```python
from build123d import *

# Parameters (mm, degrees)
SKETCH_1_R          = 1.35
EXTRUDE_1_DEPTH     = 40
EXTRUDE_2_DEPTH     = 10
SKETCH_3_W          = 36
SKETCH_3_H          = 37.441664415
SKETCH_3_R          = 11
EXTRUDE_3_DEPTH     = 5
SKETCH_4_R          = 1.8
CUT_EXTRUDE_1_DEPTH = 18
SKETCH_5_R          = 1.35
CUT_EXTRUDE_2_DEPTH = 18
CUT_EXTRUDE_START   = -5
SKETCH_6_R          = 11
CUT_EXTRUDE_3_DEPTH = 5
SKETCH_7_W          = 36
SKETCH_7_H          = 37.441664415
CUT_EXTRUDE_4_DEPTH = 5
CUT_EXTRUDE_START_2 = -12
SKETCH_8_R          = 1.35
CUT_EXTRUDE_5_DEPTH = 12
SKETCH_10_R         = 1.34
SKETCH_10_R_2       = 1.35
CUT_EXTRUDE_6_DEPTH = 8


with BuildPart() as part:
    # 草图1 → 凸台-拉伸1 (new body)
    with BuildSketch(Plane.XY):
        with BuildLine():
            Line((-10, -4), (10, -4))
            ThreePointArc((10, -4), (13.795550466, -1.262456597), (12.395858862, 3.203101671))
            Line((12.395858862, 3.203101671), (6.347732719, 7.726984491))
            Line((6.347732719, 7.726984491), (0, 7.726984491))
            Line((0, 7.726984491), (-6.347732719, 7.726984491))
            Line((-6.347732719, 7.726984491), (-12.395858862, 3.203101671))
            ThreePointArc((-12.395858862, 3.203101671), (-13.795550466, -1.262456597), (-10, -4))
        make_face()
        with Locations((10, 0)):
            Circle(SKETCH_1_R, mode=Mode.SUBTRACT)
        with Locations((-10, 0)):
            Circle(SKETCH_1_R, mode=Mode.SUBTRACT)
    extrude(amount=EXTRUDE_1_DEPTH)

    # 草图2 → 凸台-拉伸2 (add)
    with BuildSketch(Plane.XZ.offset(4)):
        Polygon((-10, 37.441664415), (-18, 37.441664415), (-18, 0), (0, 0), (10, 0), (18, 0), (18, 37.441664415), align=None)
    extrude(amount=-EXTRUDE_2_DEPTH)

    # 草图3 → 凸台-拉伸3 (add)
    with BuildSketch(Plane.XZ.offset(4)):
        with Locations((0, 18.720832208)):
            Rectangle(SKETCH_3_W, SKETCH_3_H)
        with Locations(Location((0, 16, 0), (0, 0, 270))):
            Circle(SKETCH_3_R, mode=Mode.SUBTRACT)
    extrude(amount=EXTRUDE_3_DEPTH)

    # 草图4 → 切除-拉伸1 (cut)
    with BuildSketch(Plane.XZ.offset(4)):
        with Locations(Location((0, 16, 0), (0, 0, 270))):
            Circle(SKETCH_4_R)
    extrude(amount=-CUT_EXTRUDE_1_DEPTH, mode=Mode.SUBTRACT)

    # 草图5 → 切除-拉伸2 (cut)
    with BuildSketch(Plane.XZ.offset(9)):
        with Locations(Location((-15, 16, 0), (0, 0, 270))):
            Circle(SKETCH_5_R)
        with Locations(Location((15, 16, 0), (0, 0, 270))):
            Circle(SKETCH_5_R)
    extrude(amount=-CUT_EXTRUDE_2_DEPTH, mode=Mode.SUBTRACT)

    # 草图6 → 切除-拉伸3 (cut)
    with BuildSketch(Plane.XZ.offset(4).offset(CUT_EXTRUDE_START)):
        with Locations(Location((0, 16, 0), (0, 0, 270))):
            Circle(SKETCH_6_R)
    extrude(amount=CUT_EXTRUDE_3_DEPTH, mode=Mode.SUBTRACT)

    # 草图7 → 切除-拉伸4 (cut)
    with BuildSketch(Plane.XZ.offset(9)):
        with Locations((0, 18.720832208)):
            Rectangle(SKETCH_7_W, SKETCH_7_H)
    extrude(amount=-CUT_EXTRUDE_4_DEPTH, mode=Mode.SUBTRACT)

    # 草图8 → 切除-拉伸5 (cut)
    with BuildSketch(Plane.XY.offset(37.441664415).offset(CUT_EXTRUDE_START_2)):
        with Locations((10, 0)):
            Circle(SKETCH_8_R)
        with Locations((-10, 0)):
            Circle(SKETCH_8_R)
    extrude(amount=CUT_EXTRUDE_5_DEPTH, mode=Mode.SUBTRACT)

    # 草图10 → 切除-拉伸6 (cut)
    with BuildSketch(Plane(origin=(0, 0, 0), x_dir=(-1, 0, 0), z_dir=(0, 0, -1))):
        with Locations((10, 0)):
            Circle(SKETCH_10_R)
        with Locations(Location((-10, 0, 0), (0, 0, 180))):
            Circle(SKETCH_10_R_2)
    extrude(amount=-CUT_EXTRUDE_6_DEPTH, mode=Mode.SUBTRACT)


solid = part.part
```
Here's how the part is built. I have some questions about the finished solid (model axes, mm). A direction names the side the tool comes from. Give positions to 0.01 mm unless a question says otherwise; leave off trailing zeros. Order: outer loops, then holes, each group sorted by start corner. A loop starts at its lowest first (then second) coordinate and runs counter-clockwise, first axis right, second up. Notation, with made-up numbers: (19, 50) -> (28, 50) arc R21 cw to (28, 79) -> close; hole circle Ø7 at (75.5, 72.5). An arc over 180 degrees is marked (long way). Use CSV: the item, a comma, the result in double quotes. Start each with the question number.
Item 1: Suppose I cut it at C-C (z = 30.5). List the corners of the cut face in (x, y) for me.
Item 2: I'm going to push flat-ended pins straight in: P1, Ø2.5, axis at x = 10, y = 0, coming from the -Z side; P2, Ø2, axis at x = 10, y = 0, coming from the +Z side; P3, Ø4.5, axis at x = 15.5, z = 26.5, coming from the +Y side. Where does each tip first touch, or does it pass through?
Item 3: On a 3-axis mill with a long thin cutter (end or side, diameter ignored), from which of +Z, -Z, +X, -X, +Y, -Y can I reach the whole of each face in a straight line? I mean faces 1 (the flat face through (10, 0, 8)), 2 (the cylindrical face through (13.773, -1.329, 38.703)), 3 (the cylindrical face through (-8.753, -0.517, 32.619)), 4 (the flat face through (13, 6, 19)). Say none if no direction works.
Item 4: Thinking about a two-plate mould opening in Z: for faces 5 (the flat face through (18, 1, 18)), 6 (the flat face through (10, 0, 25.442)), 7 (the cylindrical face through (16.339, 0.93, 16.176)), which applies, pulls with the +Z half, pulls with the -Z half, needs draft (parallel to the pull), parting line crosses it, or undercut?
Item 5: If I drill on probe 1 along X at (y, z) = (4, 16); probe 2 along X at (y, z) = (-1.45, 16); probe 3 along Y at (x, z) = (10, 5), over which ranges is the centre line in solid material (lowest first)? Write a range as [from, to].
Item 6: Suppose I cut it at D-D (y = 0). List the corners of the cut face in (x, z) for me, and give its area (3 significant figures).
Item 7: Suppose I cut it at B-B (x = -15). List the corners of the cut face in (y, z) for me.
Item 8: Suppose I cut it at A-A (z = 16). List the corners of the cut face in (x, y) for me.
Answer block:
1,outline,"(-18, -4) -> (18, -4) -> (18, 6) -> (8.66, 6) -> (6.35, 7.73) -> (-6.35, 7.73) -> (-8.66, 6) -> (-18, 6) -> close; hole circle Ø2.7 at (-10, 0); hole circle Ø2.7 at (10, 0)"
2,P1,"stops at z = 8"
2,P2,"stops at z = 25.44"
2,P3,"stops at y = 6"
3,face 1,"-Z"
3,face 2,"+Z, +X"
3,face 3,"+Z"
3,face 4,"+Z, -Z, +X, +Y"
4,face 5,"needs draft"
4,face 6,"pulls with the +Z half"
4,face 7,"undercut"
5,probe 1,"x = [-18, -16.35], [-13.65, -1.8], [1.8, 13.65], [16.35, 18]"
5,probe 2,"x = [-18, -16.35], [-13.65, -11], [11, 13.65], [16.35, 18]"
5,probe 3,"y = [-4, -1.35], [1.35, 6]"
6,outline,"(-18, 0) -> (-11.34, 0) -> (-11.34, 8) -> (-8.66, 8) -> (-8.66, 0) -> (8.65, 0) -> (8.65, 8) -> (11.35, 8) -> (11.35, 0) -> (18, 0) -> (18, 37.44) -> (14, 37.44) -> (14, 40) -> (11.35, 40) -> (11.35, 25.44) -> (8.65, 25.44) -> (8.65, 40) -> (-8.65, 40) -> (-8.65, 25.44) -> (-11.35, 25.44) -> (-11.35, 40) -> (-14, 40) -> (-14, 37.44) -> (-18, 37.44) -> close; hole circle Ø2.7 at (-15, 16); hole circle Ø22 at (0, 16); hole circle Ø2.7 at (15, 16)"
6,area,"906 mm^2"
7,outline,"(-4, 0) -> (6, 0) -> (6, 14.65) -> (-4, 14.65) -> close; (-4, 17.35) -> (6, 17.35) -> (6, 37.44) -> (-4, 37.44) -> close"
8,outline,"(-18, -4) -> (-16.35, -4) -> (-16.35, 6) -> (-18, 6) -> close; (-13.65, -4) -> (-11, -4) -> (-11, 1) -> (-1.8, 1) -> (-1.8, 7.73) -> (-6.35, 7.73) -> (-8.66, 6) -> (-13.65, 6) -> close; (1.8, 1) -> (11, 1) -> (11, -4) -> (13.65, -4) -> (13.65, 6) -> (8.66, 6) -> (6.35, 7.73) -> (1.8, 7.73) -> close; (16.35, -4) -> (18, -4) -> (18, 6) -> (16.35, 6) -> close"
